Drawing for the job (mm, zero at the part's lowest x, y, z). Give positions to 0.01 mm unless a question says otherwise; leave off trailing zeros. Loops run counter-clockwise (first coordinate to the right, second up) from the corner with the lowest first, then second, coordinate; pieces in that order, holes last. Notation, with made-up numbers: (77, -7) -> (104, -7) arc R10 cw to (104, 3) -> close; hole circle Ø10 at (68, -37.75). An arc over 180 degrees is marked (long way). Write item = value, one per line.
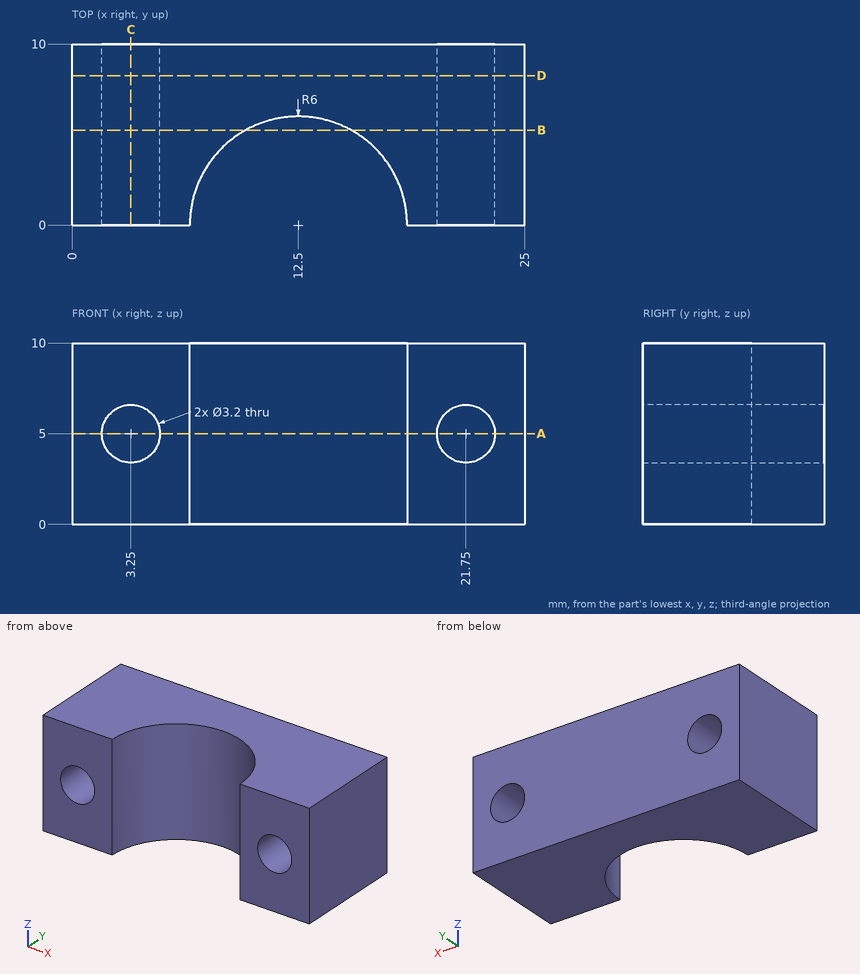
1) Slice it at D-D, the plane y = 8.25. List the corners of the cut face in (x, z), and give its area (3 significant figures).
Resolved:
outline = (0, 0) -> (25, 0) -> (25, 10) -> (0, 10) -> close; hole circle Ø3.2 at (3.25, 5); hole circle Ø3.2 at (21.75, 5)
area = 234 mm²
2) Slice it at C-C, the plane x = 3.25. List the corners of the cut face in (y, z).
Resolved:
outline = (0, 0) -> (10, 0) -> (10, 3.4) -> (0, 3.4) -> close; (0, 6.6) -> (10, 6.6) -> (10, 10) -> (0, 10) -> close
3) Slice it at B-B, the plane y = 5.25. List the corners of the cut face in (x, z).
Resolved:
outline = (0, 0) -> (9.6, 0) -> (9.6, 10) -> (0, 10) -> close; (15.4, 0) -> (25, 0) -> (25, 10) -> (15.4, 10) -> close; hole circle Ø3.2 at (3.25, 5); hole circle Ø3.2 at (21.75, 5)
4) Slice it at A-A, the plane z = 5. List the corners of the cut face in (x, y).
Resolved:
outline = (0, 0) -> (1.65, 0) -> (1.65, 10) -> (0, 10) -> close; (4.85, 0) -> (6.5, 0) arc R6 cw to (18.5, 0) -> (20.15, 0) -> (20.15, 10) -> (4.85, 10) -> close; (23.35, 0) -> (25, 0) -> (25, 10) -> (23.35, 10) -> close
5) Drill centre lines: line 1 along X through (y, z) = (6.25, 5); line 2 along X through (y, z) = (4, 6.25); line 3 along X through (y, z) = (8.25, 4.25). Where is each one in solid material? Low to high. Write a range as [from, to].
Resolved:
line_1 = [0, 1.65], [4.85, 20.15], [23.35, 25]
line_2 = [0, 2.25], [4.25, 8.03], [16.97, 20.75], [22.75, 25]
line_3 = [0, 1.84], [4.66, 20.34], [23.16, 25]
6) Drop a flat-ended pin along its axis: P1, Ø3, axis at x = 22.5, y = 7.5, coming from the -Z side. Give the stop position or say it passes through.
Resolved:
P1 = 0
